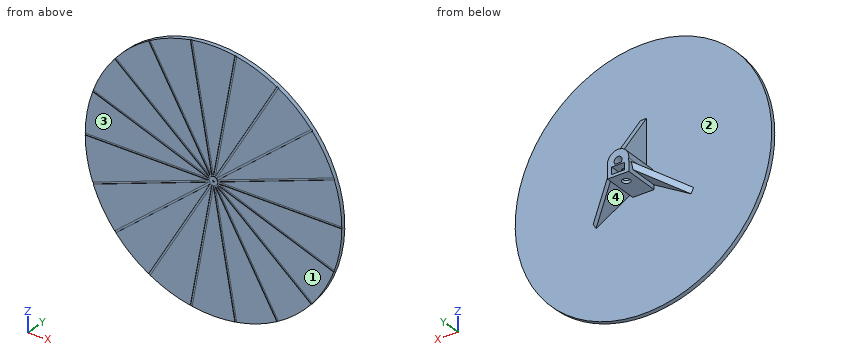
from build123d import *

# Parameters (mm, degrees)
SKETCH1_R                = 90
BOSS_EXTRUDE1_DEPTH      = 3
SKETCH2_R                = 7.5
BOSS_EXTRUDE2_DEPTH      = 25
RIB5_REACH               = 132.323
SKETCH3_WALL_W           = 306.218438134
SKETCH3_WALL_H           = 4
CIRPATTERN1_COUNT        = 3
BOSS_EXTRUDE3_DEPTH      = 4
BOSS_EXTRUDE3_DEPTH_BACK = 3
BOSS_EXTRUDE3_START      = -5
SKETCH5_W                = 15
SKETCH5_H                = 25
SKETCH5_R                = 2.75
CUT_EXTRUDE3_DEPTH       = 130.711217711
CUT_EXTRUDE3_DEPTH_BACK  = 1
SKETCH8_R                = 2.75
CUT_EXTRUDE4_DEPTH       = 8
CUT_EXTRUDE1_START       = -1
CUT_EXTRUDE1_DEPTH       = 5
SKETCH9_W                = 11.211365442
SKETCH9_H                = 11.7257459
SKETCH9_R                = 2.75
BOSS_EXTRUDE4_DEPTH      = 2
SKETCH10_W               = 9
SKETCH10_H               = 5
CUT_EXTRUDE5_DEPTH       = 10.453739
FILLET1_START            = 2
FILLET1_DEPTH            = 26
SKETCH11_R               = 3
CUT_EXTRUDE6_DEPTH       = 0.36
SKETCH12_R               = 0.6
CUT_EXTRUDE7_DEPTH       = 0.36


with BuildPart() as part:
    # Sketch1 → Boss-Extrude1 (new body)
    with BuildSketch(Plane(origin=(0, 0, 0), x_dir=(1, 0, 0), z_dir=(0, 1, 0))):
        with Locations(Location((0, 0, 0), (0, 0, 270))):
            Circle(SKETCH1_R)
    extrude(amount=BOSS_EXTRUDE1_DEPTH)

    # Sketch2 → Boss-Extrude2 (add)
    with BuildSketch(Plane(origin=(0, 3, 0), x_dir=(1, 0, 0), z_dir=(0, 1, 0))):
        with Locations(Location((0, 0, 0), (0, 0, 270))):
            Circle(SKETCH2_R)
        with BuildLine():
            Line((-2.121320344, 1.75), (2.121320344, 1.75))
            ThreePointArc((2.121320344, 1.75), (0, -2.75), (-2.121320344, 1.75))
        make_face(mode=Mode.SUBTRACT)
    extrude(amount=BOSS_EXTRUDE2_DEPTH)

    # Sketch3 wall → Rib5 (add, up to next)
    with BuildSketch(Plane(origin=(0, 13.5, 24.582023983), x_dir=(0, -0.573748677161, 0.819031412985), z_dir=(0, -0.819031412985, -0.573748677161)), mode=Mode.PRIVATE) as rib5_sk1:
        Rectangle(SKETCH3_WALL_W, SKETCH3_WALL_H)
    rib5_tool1 = extrude(rib5_sk1.sketch, amount=RIB5_REACH, mode=Mode.PRIVATE) - part.part
    rib5 = rib5_tool1.solids().sort_by_distance((0, 13.5, 24.582023983))[0]
    add(rib5)

    # CirPattern1: Rib5 ×3 about axis
    cirpattern1_axis = Axis((0, 0, 0), (0, 1, 0))
    for i in range(1, CIRPATTERN1_COUNT):
        add(rib5.rotate(cirpattern1_axis, i * 360 / CIRPATTERN1_COUNT))

    # Sketch5 → Boss-Extrude3 (add, two sides: drawn at the far end of the back side and taken through both)
    with BuildSketch(Plane.XY.offset(-1.75).offset(BOSS_EXTRUDE3_START - BOSS_EXTRUDE3_DEPTH_BACK)):
        with Locations((0, 15.5)):
            Rectangle(SKETCH5_W, SKETCH5_H)
        with Locations(Location((0, 20, 0), (0, 0, 90))):
            Circle(SKETCH5_R, mode=Mode.SUBTRACT)
    extrude(amount=BOSS_EXTRUDE3_DEPTH + BOSS_EXTRUDE3_DEPTH_BACK)

    # Sketch7 → Cut-Extrude3 (cut, two sides: drawn at the far end of the back side and taken through both)
    with BuildSketch(Plane(origin=(0, 3, 0), x_dir=(1, 0, 0), z_dir=(0, 1, 0)).offset(-CUT_EXTRUDE3_DEPTH_BACK)):
        with BuildLine():
            Line((-2.121320344, 1.75), (2.121320344, 1.75))
            ThreePointArc((2.121320344, 1.75), (0, -2.75), (-2.121320344, 1.75))
        make_face()
    extrude(amount=CUT_EXTRUDE3_DEPTH + CUT_EXTRUDE3_DEPTH_BACK, mode=Mode.SUBTRACT)

    # Sketch8 → Cut-Extrude4 (cut)
    with BuildSketch(Plane(origin=(0, 0, -9.75), x_dir=(-1, 0, 0), z_dir=(0, 0, -1))):
        with Locations(Location((0, 20, 0), (0, 0, 39.521196359))):
            Circle(SKETCH8_R)
    extrude(amount=-CUT_EXTRUDE4_DEPTH, mode=Mode.SUBTRACT)

    # Sketch4 → Cut-Extrude1 (cut)
    with BuildSketch(Plane.XY.offset(-1.75).offset(CUT_EXTRUDE1_START)):
        Polygon((0, 24.907477288), (-4.25, 22.453738644), (-4.25, 17.546261356), (0, 15.092522712), (4.25, 17.546261356), (4.25, 22.453738644), align=None)
    extrude(amount=-CUT_EXTRUDE1_DEPTH, mode=Mode.SUBTRACT)

    # Sketch9 → Boss-Extrude4 (add)
    with BuildSketch(Plane(origin=(0, 0, -9.75), x_dir=(-1, 0, 0), z_dir=(0, 0, -1))):
        with Locations((0, 20)):
            Rectangle(SKETCH9_W, SKETCH9_H)
        with Locations(Location((0, 20, 0), (0, 0, 180))):
            Circle(SKETCH9_R, mode=Mode.SUBTRACT)
    extrude(amount=-BOSS_EXTRUDE4_DEPTH)

    # Sketch10 → Cut-Extrude5 (cut)
    with BuildSketch(Plane(origin=(0, 28, 0), x_dir=(1, 0, 0), z_dir=(0, 1, 0))):
        with Locations((0, 5.25)):
            Rectangle(SKETCH10_W, SKETCH10_H)
    extrude(amount=-CUT_EXTRUDE5_DEPTH, mode=Mode.SUBTRACT)

    # Fillet1: read off the stored shape, not the designer's step
    # Fillet1 outline → Fillet1 (add)
    with BuildSketch(Plane(origin=(0, 0, 0), x_dir=(1, 0, 0), z_dir=(0, 1, 0)).offset(FILLET1_START)):
        with BuildLine():
            ThreePointArc((-7.46988647, 0.671413522), (-7.29814404, 1.728321024), (-6.977642868, 2.75))
            Line((-6.977642868, 2.75), (-7.5, 2.75))
            ThreePointArc((-7.5, 2.75), (-7.430784372, 1.711491388), (-7.46988647, 0.671413522))
        make_face()
        with BuildLine():
            Line((7.5, 2.75), (6.977642868, 2.75))
            ThreePointArc((6.977642868, 2.75), (7.29814404, 1.728321024), (7.46988647, 0.671413522))
            ThreePointArc((7.46988647, 0.671413522), (7.430784372, 1.711491388), (7.5, 2.75))
        make_face()
    extrude(amount=FILLET1_DEPTH)

    # Sketch11 → Cut-Extrude6 (cut)
    with BuildSketch(Plane.XZ):
        with BuildLine():
            Line((-89.997579967, 0.66), (-3.743046001, 0.66))
            Line((-3.743046001, 0.66), (-84.795795079, 30.16078807))
            ThreePointArc((-84.795795079, 30.16078807), (-84.572335871, 30.781812899), (-84.344328489, 31.401182329))
            Line((-84.344328489, 31.401182329), (-3.291579412, 1.900394259))
            Line((-3.291579412, 1.900394259), (-69.366385851, 57.343739972))
            ThreePointArc((-69.366385851, 57.343739972), (-68.943999881, 57.850884872), (-68.517906206, 58.354918637))
            Line((-68.517906206, 58.354918637), (-2.443099767, 2.911572924))
            Line((-2.443099767, 2.911572924), (-45.57036675, 77.610190531))
            ThreePointArc((-45.57036675, 77.610190531), (-45, 77.942286341), (-44.427213217, 78.270190531))
            Line((-44.427213217, 78.270190531), (-1.299946234, 3.571572924))
            Line((-1.299946234, 3.571572924), (-16.277888873, 88.515706707))
            ThreePointArc((-16.277888873, 88.515706707), (-15.62833599, 88.632697771), (-14.977942639, 88.744922302))
            Line((-14.977942639, 88.744922302), (0, 3.800788519))
            Line((0, 3.800788519), (14.977942639, 88.744922302))
            ThreePointArc((14.977942639, 88.744922302), (15.62833599, 88.632697771), (16.277888873, 88.515706707))
            Line((16.277888873, 88.515706707), (1.299946234, 3.571572924))
            Line((1.299946234, 3.571572924), (44.427213217, 78.270190531))
            ThreePointArc((44.427213217, 78.270190531), (45, 77.942286341), (45.57036675, 77.610190531))
            Line((45.57036675, 77.610190531), (2.443099767, 2.911572924))
            Line((2.443099767, 2.911572924), (68.517906206, 58.354918637))
            ThreePointArc((68.517906206, 58.354918637), (68.943999881, 57.850884872), (69.366385851, 57.343739972))
            Line((69.366385851, 57.343739972), (3.291579412, 1.900394259))
            Line((3.291579412, 1.900394259), (84.344328489, 31.401182329))
            ThreePointArc((84.344328489, 31.401182329), (84.572335871, 30.781812899), (84.795795079, 30.16078807))
            Line((84.795795079, 30.16078807), (3.743046001, 0.66))
            Line((3.743046001, 0.66), (89.997579967, 0.66))
            ThreePointArc((89.997579967, 0.66), (90, 0), (89.997579967, -0.66))
            Line((89.997579967, -0.66), (3.743046001, -0.66))
            Line((3.743046001, -0.66), (84.795795079, -30.16078807))
            ThreePointArc((84.795795079, -30.16078807), (84.572335871, -30.781812899), (84.344328489, -31.401182329))
            Line((84.344328489, -31.401182329), (3.291579412, -1.900394259))
            Line((3.291579412, -1.900394259), (69.366385851, -57.343739972))
            ThreePointArc((69.366385851, -57.343739972), (68.943999881, -57.850884872), (68.517906206, -58.354918637))
            Line((68.517906206, -58.354918637), (2.443099767, -2.911572924))
            Line((2.443099767, -2.911572924), (45.57036675, -77.610190531))
            ThreePointArc((45.57036675, -77.610190531), (45, -77.942286341), (44.427213217, -78.270190531))
            Line((44.427213217, -78.270190531), (1.299946234, -3.571572924))
            Line((1.299946234, -3.571572924), (16.277888873, -88.515706707))
            ThreePointArc((16.277888873, -88.515706707), (15.62833599, -88.632697771), (14.977942639, -88.744922302))
            Line((14.977942639, -88.744922302), (0, -3.800788519))
            Line((0, -3.800788519), (-14.977942639, -88.744922302))
            ThreePointArc((-14.977942639, -88.744922302), (-15.62833599, -88.632697771), (-16.277888873, -88.515706707))
            Line((-16.277888873, -88.515706707), (-1.299946234, -3.571572924))
            Line((-1.299946234, -3.571572924), (-44.427213217, -78.270190531))
            ThreePointArc((-44.427213217, -78.270190531), (-45, -77.942286341), (-45.57036675, -77.610190531))
            Line((-45.57036675, -77.610190531), (-2.443099767, -2.911572924))
            Line((-2.443099767, -2.911572924), (-68.517906206, -58.354918637))
            ThreePointArc((-68.517906206, -58.354918637), (-68.943999881, -57.850884872), (-69.366385851, -57.343739972))
            Line((-69.366385851, -57.343739972), (-3.291579412, -1.900394259))
            Line((-3.291579412, -1.900394259), (-84.344328489, -31.401182329))
            ThreePointArc((-84.344328489, -31.401182329), (-84.572335871, -30.781812899), (-84.795795079, -30.16078807))
            Line((-84.795795079, -30.16078807), (-3.743046001, -0.66))
            Line((-3.743046001, -0.66), (-89.997579967, -0.66))
            ThreePointArc((-89.997579967, -0.66), (-90, 0), (-89.997579967, 0.66))
        make_face()
        with Locations(Location((0, 0, 0), (0, 0, 270))):
            Circle(SKETCH11_R, mode=Mode.SUBTRACT)
    extrude(amount=-CUT_EXTRUDE6_DEPTH, mode=Mode.SUBTRACT)

    # Sketch12 → Cut-Extrude7 (cut)
    with BuildSketch(Plane.XZ):
        with Locations(Location((0, 0, 0), (0, 0, 270))):
            Circle(SKETCH12_R)
    extrude(amount=-CUT_EXTRUDE7_DEPTH, mode=Mode.SUBTRACT)


solid = part.part
Geometry check sheet. Reference: the model listing, model coordinates, mm. Face numbers are marked on the shaded views. A direction names the side the tool comes from. Give positions to 0.01 mm unless a question says otherwise; leave off trailing zeros. Order: outer loops, then holes, each group sorted by start corner. A loop starts at its lowest first (then second) coordinate and runs counter-clockwise, first axis right, second up.
1. Sectioned sample at C-C (z = -44.5). Record the boundary of the cut face in (x, y).
Completed:
outline: (-78.23, 0) - (-54.06, 0) - (-54.06, 0.36) - (-52.01, 0.36) - (-52.01, 0) - (-26.45, 0) - (-26.45, 0.36) - (-24.93, 0.36) - (-24.93, 0) - (-8.52, 0) - (-8.52, 0.36) - (-7.18, 0.36) - (-7.18, 0) - (7.18, 0) - (7.18, 0.36) - (8.52, 0.36) - (8.52, 0) - (24.93, 0) - (24.93, 0.36) - (26.45, 0.36) - (26.45, 0) - (52.01, 0) - (52.01, 0.36) - (54.06, 0.36) - (54.06, 0) - (78.23, 0) - (78.23, 3) - (-78.23, 3) - close
2. Sectioned sample at A-A (z = 70). Record the boundary of the cut face in (x, y), then the cut area to 3 significant figures.
Completed:
outline: (-56.57, 0) - (-41.18, 0) - (-41.18, 0.36) - (-39.65, 0.36) - (-39.65, 0) - (-13.01, 0) - (-13.01, 0.36) - (-11.67, 0.36) - (-11.67, 0) - (11.67, 0) - (11.67, 0.36) - (13.01, 0.36) - (13.01, 0) - (39.65, 0) - (39.65, 0.36) - (41.18, 0.36) - (41.18, 0) - (56.57, 0) - (56.57, 3) - (-56.57, 3) - close
area: 337 mm2
3. Sectioned sample at D-D (x = 63). Record the boundary of the cut face in (y, z), then the cut area to 3 significant figures.
Completed:
outline: (0, -64.27) - (3, -64.27) - (3, 64.27) - (0, 64.27) - (0, 53.72) - (0.36, 53.72) - (0.36, 52) - (0, 52) - (0, 23.63) - (0.36, 23.63) - (0.36, 22.23) - (0, 22.23) - (0, 0.66) - (0.36, 0.66) - (0.36, -0.66) - (0, -0.66) - (0, -22.23) - (0.36, -22.23) - (0.36, -23.63) - (0, -23.63) - (0, -52) - (0.36, -52) - (0.36, -53.72) - (0, -53.72) - close
area: 383 mm2
4. Depth check by flat-ended pin: pin 1 (2.5 mm diameter, centred on x = 0.5, y = 20, fed in from -Z); pin 2 (5 mm diameter, centred on x = 0, y = 20, fed in from +Z); pin 3 (1 mm diameter, centred on y = 23, z = 11, fed in from -X). Enter the tip coordinate at first touch or a pass-through.
Completed:
pin 1: stops at z = 2.12
pin 2: stops at z = 18.87
pin 3: stops at x = -2
5. Access from +Z, -Z, +X, -X, +Y, -Y to the whole of each face (thin tool, end or side, straight path). Record for the marked faces 1 and 2.
Completed:
face 1: +Z, -Z, +X, -X, -Y
face 2: +Y
6. Scan lines: line 1 (X direction, y = 13.25, z = 0); line 2 (X direction, y = 20, z = -8.45); line 3 (X direction, y = 20, z = -9). Record each from-to range of solid material in increasing order.
Completed:
line 1: x = -7.5 to -2.75, 2.75 to 7.5
line 2: x = -12.79 to -10.64, -7.5 to -2.75, 2.75 to 7.5, 10.64 to 12.79
line 3: x = -12.47 to -11.59, -7.5 to -2.75, 2.75 to 7.5, 11.59 to 12.47
7. Draft check along Z on the marked faces 3 and 4. Enter one of: pulls with the +Z half, pulls with the -Z half, needs draft (parallel to the pull), parting line crosses it, or undercut.
Completed:
face 3: needs draft
face 4: pulls with the -Z half
